from build123d import *

# Parameters (mm, degrees)
SKETCH1_R           = 2.4
BOSS_EXTRUDE3_DEPTH = 3.9
SKETCH3_R           = 3.05
CUT_EXTRUDE16_DEPTH = 0.8
SKETCH4_R           = 3.05
CUT_EXTRUDE17_DEPTH = 0.8


with BuildPart() as part:
    # Sketch1 → Boss-Extrude3 (new body)
    with BuildSketch(Plane(origin=(0, 0, 0), x_dir=(1, 0, 0), z_dir=(0, 1, 0))):
        with BuildLine():
            Line((-8.030145899, -3.65), (8.039854101, -3.65))
            ThreePointArc((8.039854101, -3.65), (10.620793852, -2.580939751), (11.689854101, 0))
            Line((11.689854101, 0), (11.689854101, 32.1))
            ThreePointArc((11.689854101, 32.1), (9.706187522, 35.407989059), (5.862167957, 35.08980939))
            ThreePointArc((5.862167957, 35.08980939), (-6.996855856, 21.685482921), (-11.680145899, 3.710576637))
            Line((-11.680145899, 3.710576637), (-11.680145899, 0))
            ThreePointArc((-11.680145899, 0), (-10.611085651, -2.580939751), (-8.030145899, -3.65))
        make_face()
        with Locations((0.004854101, 0)):
            Circle(SKETCH1_R, mode=Mode.SUBTRACT)
        with Locations((8.039854101, 24.12)):
            Circle(SKETCH1_R, mode=Mode.SUBTRACT)
        with Locations((8.039854101, 16.08)):
            Circle(SKETCH1_R, mode=Mode.SUBTRACT)
        with Locations((8.039854101, 8.04)):
            Circle(SKETCH1_R, mode=Mode.SUBTRACT)
        with BuildLine():
            Line((-8.025815842, 3.649998716), (4.389854101, 3.649998716))
            Line((4.389854101, 3.649998716), (4.389854101, 29.443552649))
            ThreePointArc((4.389854101, 29.443552649), (-4.761047259, 17.963414157), (-8.025815842, 3.649998716))
        make_face(mode=Mode.SUBTRACT)
        Polygon((-8.930145899, 0.9), (-10.430145899, 0.9), (-10.430145899, -0.9), (-8.930145899, -0.9), (-8.930145899, -2.4), (-7.130145899, -2.4), (-7.130145899, -0.9), (-5.630145899, -0.9), (-5.630145899, 0.9), (-7.130145899, 0.9), (-7.130145899, 2.4), (-8.930145899, 2.4), align=None, mode=Mode.SUBTRACT)
        Polygon((10.439854101, -0.9), (8.939854101, -0.9), (8.939854101, -2.4), (7.139854101, -2.4), (7.139854101, -0.9), (5.639854101, -0.9), (5.639854101, 0.9), (7.139854101, 0.9), (7.139854101, 2.4), (8.939854101, 2.4), (8.939854101, 0.9), (10.439854101, 0.9), align=None, mode=Mode.SUBTRACT)
        Polygon((5.639854101, 33.06), (7.139854101, 33.06), (7.139854101, 34.56), (8.939854101, 34.56), (8.939854101, 33.06), (10.439854101, 33.06), (10.439854101, 31.26), (8.939854101, 31.26), (8.939854101, 29.76), (7.139854101, 29.76), (7.139854101, 31.26), (5.639854101, 31.26), align=None, mode=Mode.SUBTRACT)
    extrude(amount=BOSS_EXTRUDE3_DEPTH)

    # Sketch3 → Cut-Extrude16 (cut)
    with BuildSketch(Plane(origin=(0, 3.9, 0), x_dir=(1, 0, 0), z_dir=(0, 1, 0))):
        with Locations((0.004854101, 0)):
            Circle(SKETCH3_R)
        with Locations((8.039854101, 8.04)):
            Circle(SKETCH3_R)
        with Locations((8.039854101, 16.08)):
            Circle(SKETCH3_R)
        with Locations((8.039854101, 24.12)):
            Circle(SKETCH3_R)
    extrude(amount=-CUT_EXTRUDE16_DEPTH, mode=Mode.SUBTRACT)

    # Sketch4 → Cut-Extrude17 (cut)
    with BuildSketch(Plane.XZ):
        Circle(SKETCH4_R)
        with Locations((8.039854101, -8.04)):
            Circle(SKETCH4_R)
        with Locations((8.039854101, -16.08)):
            Circle(SKETCH4_R)
        with Locations((8.039854101, -24.12)):
            Circle(SKETCH4_R)
    extrude(amount=-CUT_EXTRUDE17_DEPTH, mode=Mode.SUBTRACT)


solid = part.part
Build history of the part. All positions in model axes, mm. A direction names the side the tool comes from. Coordinates: 2 decimals unless noted, no trailing zeros. Order: outer loops, then holes, each group sorted by start corner. A loop starts at its lowest first (then second) coordinate and runs counter-clockwise, first axis right, second up. Notation, with made-up numbers: (30, 31.25) - (55, 31.25) arc R33 cw to (55, 66.25) - close; hole circle Ø3 at (20, 26). An arc over 180 degrees is marked (long way). Write item = value, one per line. Start each with the question number.
1) Flat gauge pins, fed straight in: pin 1 Ø8 at (x, z) = (8.04, -24.12) entering from -Y; pin 2 Ø1.5 at (x, y) = (-5.5, 2.5) entering from -Z; pin 3 Ø0.8 at (y, z) = (2, 1.5) entering from +X; pin 4 Ø1.2 at (x, y) = (6.5, 1) entering from -Z. Where does each tip first touch, or does it go through?
2) Two-plate mould, pull along X, no slides. Class faces 4 (the face through (8.94, 2, -34)), 5 (the face through (5, 3.9, -12)): pulls with the +X half, pulls with the -X half, needs draft (parallel to the pull), parting line crosses it, or undercut.
3) Wall check: line 1 along X through (y, z) = (2.8, -16.5); line 2 along X through (y, z) = (0.6, -4); line 3 along Z through (x, y) = (-2.75, 0.25). Give the ranges that are in metal, low to high. Write a range as from..to.
4) Saw through at A-A on z = -24.12. Write the cut outline in (x, y).
5) Saw through at C-C on y = 1.85. Count the separate pieces of the cut face and the enclosed holes in it, then the cut area to 3 significant figures.
6) 3-axis set-ups, long thin cutter, end or side, ignore diameter. For faces 1 (the face through (-8.93, 2, -2)), 2 (the face through (10.857, 3.506, -6.872)), 3 (the face through (9.68, 0.39, -13.51)): which of +Z, -Z, +X, -X, +Y, -Y reach the whole face in a straight line?
7) Saw through at B-B on x = 0. Write the cut outline in (y, z), then the cut area to 3 significant figures.
8) Saw through at D-D on x = -4.5. Write the cut outline in (y, z).
From the geometry:
q1.pin_1 = 0
q1.pin_2 = -25.22
q1.pin_3 = 11.52
q1.pin_4 = -35.69
q2.face_4 = undercut
q2.face_5 = needs draft
q3.line_1 = -9.39..-5.42, 4.39..5.68, 10.4..11.69
q3.line_2 = -11.68..-8.02, 4.39..11.69
q3.line_3 = -27.76..-21.55, -3.65..-1.32, 1.32..3.65
q4.outline = (-5.51, 0) - (-0.91, 0) - (-0.91, 3.9) - (-5.51, 3.9) - close; (4.39, 0) - (4.99, 0) - (4.99, 0.8) - (5.64, 0.8) - (5.64, 3.1) - (4.99, 3.1) - (4.99, 3.9) - (4.39, 3.9) - close; (10.44, 0.8) - (11.09, 0.8) - (11.09, 0) - (11.69, 0) - (11.69, 3.9) - (11.09, 3.9) - (11.09, 3.1) - (10.44, 3.1) - close
q5.separate_pieces = 1
q5.enclosed_holes = 8
q5.area = 401 mm^2
q6.face_1 = +Y, -Y
q6.face_2 = +Y
q6.face_3 = -Y
q7.outline = (0, -30.62) - (3.9, -30.62) - (3.9, -25.22) - (0, -25.22) - close; (0, -3.65) - (3.9, -3.65) - (3.9, -3.05) - (3.1, -3.05) - (3.1, -2.4) - (0.8, -2.4) - (0.8, -3.05) - (0, -3.05) - close; (0, 3.05) - (0.8, 3.05) - (0.8, 2.4) - (3.1, 2.4) - (3.1, 3.05) - (3.9, 3.05) - (3.9, 3.65) - (0, 3.65) - close
q7.area = 28.7 mm^2
q8.outline = (0, -25.56) - (3.9, -25.56) - (3.9, -18.49) - (0, -18.49) - close; (0, -3.65) - (3.9, -3.65) - (3.9, 3.65) - (0, 3.65) - close
